The model under review builds one solid part; all positions refer to its coordinate system, in mm. Coordinates: 2 decimals unless noted, no trailing zeros. Write each loop counter-clockwise with the first axis right and the second up, starting at its lowest first coordinate (ties: lowest second). Pieces come first, ordered by that corner, then holes. Notation, with made-up numbers: (20, 87) - (35, 87) arc R10 ccw to (35, 101) - close; hole circle Ø2 at (11.5, 80.5). An arc over 180 degrees is marked (long way). Put each result on its own line as item: value. Start each with the question number.
Item 1: For pin 1 (2.5 mm diameter, centred on x = -325.3, y = 338.67, fed in from +Z); pin 2 (1.5 mm diameter, centred on x = -303, z = 1.5, fed in from +Y), all flat-tipped, find the tip position at first contact; note any pin that passes through.
Item 2: To check wall thickness, follow L1, parallel to Y at x = -307, z = 0.75; L2, parallel to X at y = 255, z = 1.05; L3, parallel to Y at x = -190, z = 1.85. State the ranges of each line that lie inside material, in increasing order. Write a range as [from, to].
Item 3: Consider section B-B on z = 0.45. State how many separate pieces and enclosed holes the cut face has, then the cut area to 3 significant figures.
Item 4: Consider section A-A on x = -241.5. Give the boundary of the cut face in (y, z), then the cut area to 3 significant figures.
Autodesk Inventor part; units mm, degrees
ref_plane "YZ Plane" through (0, 0, 0) normal (1, 0, 0) x (0, 1, 0)
ref_plane "XZ Plane" through (0, 0, 0) normal (0, 1, 0) x (-1, 0, 0)
ref_plane "XY Plane" through (0, 0, 0) normal (0, 0, 1) x (1, 0, 0)
sketch "Эскиз1" plane through (0, 0, 0) normal (0, 0, 1) x (1, 0, 0)
  circle A0 centre (10.6994, 67.6713) radius 1.5
  circle A1 centre (10.6994, 364.6713) radius 1.5
  circle A2 centre (-348.3006, 364.6713) radius 1.5
  circle A3 centre (-348.3006, 67.6713) radius 1.5
  line L0 (-355.8006, 370.6713) -> (18.1994, 370.6713)
  line L1 (18.1994, 370.6713) -> (18.1994, 53.6713)
  line L2 (18.1994, 53.6713) -> (-355.8006, 53.6713)
  line L3 (-355.8006, 53.6713) -> (-355.8006, 370.6713)
  point P0 (18.1994, 53.6713)
  dimension "d4" = 374
  dimension "d6" = 317
  dimension "d7" = 14
  dimension "d40" = 7.5
  dimension "d41" = 297
  dimension "d42" = 7.5
  dimension "d43" = 7.5
  dimension "d44" = 297
  dimension "d45" = 6
  dimension "d46" = 359
  dimension "d47" = 14
  dimension "d48" = 359
extrude "Выдавливание1" add sketch "Эскиз1" along normal blind 3
sketch "Эскиз3" plane through (0, 0, 3) normal (0, 0, 1) x (1, 0, 0)
  circle A0 centre (10.6994, 282.6713) radius 3.75
  circle A1 centre (10.6994, 319.6713) radius 3.75
  circle A2 centre (-348.3006, 321.6713) radius 2
  circle A3 centre (-348.3006, 254.6713) radius 2
  circle A4 centre (-345.3006, 137.6713) radius 1.5
  point P0 (0, 0)
sketch "Эскиз4" plane through (0, 0, 3) normal (0, 0, 1) x (1, 0, 0)
  circle A0 centre (-168.3006, 372.6713) radius 1.5
  line L0 (-179.3006, 370.6713) -> (-175.8006, 378.6713)
  line L1 (-175.8006, 378.6713) -> (-160.8006, 378.6713)
  line L2 (-160.8006, 378.6713) -> (-157.3006, 370.6713)
  line L3 (18.1994, 370.6713) -> (-355.8006, 370.6713)
  line L4 (-168.3006, 372.6713) -> (-168.3006, 378.6713)
  point P0 (0, 0)
  dimension "d49" = 8
  dimension "d50" = 22
  dimension "d51" = 15
extrude "Выдавливание3" add sketch "Эскиз4" against normal blind 3
fillet "Сопряжение1" radius 5 4 edges at (-179.3006, 370.6713, 1.5) (-157.3006, 370.6713, 1.5) (-160.8006, 378.6713, 1.5) (-175.8006, 378.6713, 1.5)
fillet "Сопряжение2" radius 5 4 edges at (-355.8006, 370.6713, 1.5) (18.1994, 370.6713, 1.5) (18.1994, 53.6713, 1.5) (-355.8006, 53.6713, 1.5)
sketch "Эскиз5" plane through (0, 0, 3) normal (0, 0, 1) x (1, 0, 0)
  line L0 (-332.3006, 327.1713) -> (-287.3006, 327.1713)
  line L1 (-287.3006, 327.1713) -> (-287.3006, 282.1713)
  line L2 (-287.3006, 282.1713) -> (-332.3006, 282.1713)
  line L3 (-332.3006, 282.1713) -> (-332.3006, 327.1713)
  line L4 (-355.8006, 365.6713) -> (-355.8006, 58.6713)
  line L5 (-182.5707, 370.6713) -> (-350.8006, 370.6713)
  line L6 (-312.3006, 370.6713) -> (-292.3006, 370.6713)
  line L7 (-292.3006, 370.6713) -> (-292.3006, 349.1713)
  line L8 (-292.3006, 349.1713) -> (-312.3006, 349.1713)
  line L9 (-312.3006, 349.1713) -> (-312.3006, 370.6713)
  circle A0 centre (-335.8006, 238.6713) radius 4.95
  line L10 (-333.3006, 213.1713) -> (-320.3006, 213.1713)
  line L11 (-320.3006, 213.1713) -> (-320.3006, 203.1713)
  line L12 (-320.3006, 203.1713) -> (-333.3006, 203.1713)
  line L13 (-333.3006, 203.1713) -> (-333.3006, 213.1713)
  circle A1 centre (-330.4506, 196.6713) radius 1.6
  circle A2 centre (-323.1506, 196.6713) radius 1.6
  line L14 (-330.4506, 196.6713) -> (-323.1506, 196.6713)
  line L15 (-326.8006, 203.1713) -> (-326.8006, 196.6713)
  circle A3 centre (-162.8006, 142.6713) radius 1.6
  line L16 (18.1994, 58.6713) -> (18.1994, 365.6713)
  line L17 (-350.8006, 53.6713) -> (13.1994, 53.6713)
  line L18 (-173.8006, 132.1713) -> (-173.8006, 123.1713) construction
  line L19 (-175.3006, 132.1713) -> (-175.3006, 123.1713)
  line L20 (-172.3006, 123.1713) -> (-172.3006, 132.1713)
  arc A4 (-172.3006, 132.1713) -> (-175.3006, 132.1713) centre (-173.8006, 132.1713) ccw
  arc A5 (-175.3006, 123.1713) -> (-172.3006, 123.1713) centre (-173.8006, 123.1713) ccw
  line L21 (-151.8006, 132.1713) -> (-151.8006, 123.1713) construction
  line L22 (-153.3006, 132.1713) -> (-153.3006, 123.1713)
  line L23 (-150.3006, 123.1713) -> (-150.3006, 132.1713)
  arc A6 (-150.3006, 132.1713) -> (-153.3006, 132.1713) centre (-151.8006, 132.1713) ccw
  arc A7 (-153.3006, 123.1713) -> (-150.3006, 123.1713) centre (-151.8006, 123.1713) ccw
  line L24 (-162.8006, 142.6713) -> (-162.8006, 102.5696) construction
  line L25 (-173.8006, 127.6713) -> (-151.8006, 127.6713) construction
  circle A8 centre (-346.3006, 134.6713) radius 1.6
  line L26 (-335.3006, 132.1713) -> (-335.3006, 123.1713)
  line L27 (-336.8006, 132.1713) -> (-336.8006, 123.1713)
  line L28 (-333.8006, 123.1713) -> (-333.8006, 132.1713)
  arc A9 (-333.8006, 132.1713) -> (-336.8006, 132.1713) centre (-335.3006, 132.1713) ccw
  arc A10 (-336.8006, 123.1713) -> (-333.8006, 123.1713) centre (-335.3006, 123.1713) ccw
  circle A11 centre (-334.3006, 349.1713) radius 1.45
  circle A12 centre (-325.3006, 338.6713) radius 1.45
  circle A13 centre (10.6994, 319.6713) radius 3.75 construction
  circle A14 centre (10.6994, 282.6713) radius 3.75 construction
  circle A15 centre (10.6994, 319.6713) radius 4.75
  circle A16 centre (10.6994, 282.6713) radius 4.75
  point P0 (0, 0)
  point P1 (-335.3006, 127.6713)
  dimension "d56" = 68.5
  dimension "d57" = 45
  dimension "d58" = 45
  dimension "d59" = 23.5
  dimension "d60" = 43.5
  dimension "d61" = 21.5
  dimension "d62" = 20
  dimension "d63" = 43.5
  dimension "d64" = 20
  dimension "d65" = 132
  dimension "d66" = 9.9
  dimension "d67" = 13
  dimension "d68" = 10
  dimension "d69" = 157.5
  dimension "d70" = 22.5
  dimension "d71" = 3.2
  dimension "d72" = 3.2
  dimension "d73" = 10.5
  dimension "d74" = 6.5
  dimension "d75" = 7.3
  dimension "d76" = 193
  dimension "d77" = 181
  dimension "d78" = 89
  dimension "d79" = 3.2
  dimension "d80" = 22
  dimension "d81" = 12
  dimension "d82" = 3
  dimension "d83" = 3
  dimension "d84" = 12
  dimension "d85" = 25
  dimension "d86" = 68
  dimension "d87" = 3.2
  dimension "d88" = 9.5
  dimension "d89" = 81
  dimension "d90" = 3
  dimension "d91" = 68
  dimension "d92" = 19
  dimension "d93" = 12
  dimension "d94" = 2.9
  dimension "d95" = 2.9
  dimension "d96" = 21.5
  dimension "d97" = 21.5
  dimension "d98" = 32
  dimension "d99" = 30.5
  dimension "d100" = 9.5
  dimension "d101" = 9.5
extrude "Выдавливание4" cut sketch "Эскиз5" against normal blind 10
fillet "Сопряжение3" radius 2 12 edges at (-312.3006, 370.6713, 1.5) (-292.3006, 370.6713, 1.5) (-312.3006, 349.1713, 1.5) (-292.3006, 349.1713, 1.5) (-332.3006, 327.1713, 1.5) (-287.3006, 327.1713, 1.5) (-287.3006, 282.1713, 1.5) (-332.3006, 282.1713, 1.5) (-333.3006, 203.1713, 1.5) (-333.3006, 213.1713, 1.5) (-320.3006, 213.1713, 1.5) (-320.3006, 203.1713, 1.5)
sketch "Эскиз6" plane through (0, 0, 3) normal (0, 0, 1) x (1, 0, 0)
  circle A0 centre (-348.3006, 335.6713) radius 2
  circle A1 centre (-348.3006, 282.6713) radius 2
  circle A2 centre (-348.3006, 254.6713) radius 2
  circle A3 centre (-348.3006, 321.6713) radius 2
  line L0 (-359.8006, 317.6713) -> (-359.8006, 321.6713)
  point P0 (0, 0)
  dimension "d107" = 67
extrude "Выдавливание5" cut sketch "Эскиз6" against normal blind 10 contours A2 | A3
properties part number "боковая  панель"
Report:
1. pin 1: through
1. pin 2: y = 349.17
2. L1: [53.67, 282.17], [327.17, 349.17]
2. L2: [-355.8, -350.27], [-346.33, 18.2]
2. L3: [53.67, 370.67]
3. separate pieces: 1
3. enclosed holes: 21
3. area: 116,000 mm²
4. outline: (53.67, 0) - (370.67, 0) - (370.67, 3) - (53.67, 3) - close
4. area: 951 mm²
